from build123d import *

# Parameters (mm, degrees)
BOSS_EXTRUDE1_DEPTH = 184.15
FILLET1_R           = 3.175
FILLET2_R           = 6.35
SKETCH2_R           = 2.4638
CUT_EXTRUDE1_DEPTH  = 39.1
SKETCH3_R           = 2.4638
CUT_EXTRUDE2_DEPTH  = 39.1
LPATTERN1_COUNT     = 4
LPATTERN1_PITCH     = 101.6


with BuildPart() as part:
    # Sketch1 → Boss-Extrude1 (new body, symmetric)
    with BuildSketch(Plane(origin=(0, 0, 0), x_dir=(0, 0, -1), z_dir=(1, 0, 0))):
        Polygon((0, 38.1), (0, 0), (-38.1, 0), (-38.1, 3.175), (-3.175, 3.175), (-3.175, 38.1), align=None)
    extrude(amount=BOSS_EXTRUDE1_DEPTH, both=True)

    # Fillet1
    fillet1_edges = [part.edges().sort_by_distance(p)[0] for p in [
        (0, 3.175, 3.175),
    ]]
    fillet(fillet1_edges, radius=FILLET1_R)

    # Fillet2
    fillet2_edges = [part.edges().sort_by_distance(p)[0] for p in [
        (0, 0, 0),
    ]]
    fillet(fillet2_edges, radius=FILLET2_R)

    # Sketch2 → Cut-Extrude1 (cut, through all)
    with BuildSketch(Plane(origin=(0, 0, 0), x_dir=(-1, 0, 0), z_dir=(0, 0, -1))):
        with Locations((152.4, 19.05)):
            Circle(SKETCH2_R)
    cut_extrude1 = extrude(amount=-CUT_EXTRUDE1_DEPTH, mode=Mode.SUBTRACT)

    # Sketch3 → Cut-Extrude2 (cut, through all)
    with BuildSketch(Plane.XZ):
        with Locations((-152.4, 19.05)):
            Circle(SKETCH3_R)
    cut_extrude2 = extrude(amount=-CUT_EXTRUDE2_DEPTH, mode=Mode.SUBTRACT)

    # LPattern1: Cut-Extrude1, Cut-Extrude2 ×4
    with Locations(*[(i * LPATTERN1_PITCH, 0, 0) for i in range(1, LPATTERN1_COUNT)]):
        add(cut_extrude1, mode=Mode.SUBTRACT)
        add(cut_extrude2, mode=Mode.SUBTRACT)


solid = part.part
Can you work these out from the model? Positions are in its coordinate system, mm. A direction names the side the tool comes from. Coordinates: 2 decimals unless noted, no trailing zeros. Order: outer loops, then holes, each group sorted by start corner. A loop starts at its lowest first (then second) coordinate and runs counter-clockwise, first axis right, second up. Notation, with made-up numbers: (-26.5, 48.25) - (20.5, 48.25) arc R20 ccw to (20.5, 56.25) - close; hole circle Ø4 at (-20, 65.5). An arc over 180 degrees is marked (long way). Answer as a JSON object with one key per item and string values. Group by question number.
Q1. On a 3-axis mill with a long thin cutter (end or side, diameter ignored), from which of +Z, -Z, +X, -X, +Y, -Y can I reach the whole of each face in a straight line? I mean faces 1 (the face through (3, 3.175, 22)), 2 (the face through (-2.58, 1.81, 1.91)). Say none if no direction works.
Q2. Imagine slicing it at B-B (z = 11.5). Please give me the cut outline in (x, y) (3 decimals), and give its area (3 significant figures).
Q3. I need wall thicknesses on line 1 (X direction, y = 19, z = 2); line 2 (Y direction, x = 1, z = 20) (3 decimals); line 3 (X direction, y = 2.5, z = 18). Which ranges of each line are inside material? Lowest first, please. Write a range as from..to.
Q4. Imagine slicing it at A-A (x = 95.5). Please give me the cut outline in (y, z) (3 decimals), and give its area (3 significant figures).
Q5. Will these pins go through, and if not, where does the flat tip stop? P1, Ø6.5, axis at x = 152.4, y = 19.05, coming from the +Z side (3 decimals); P2, Ø6.5, axis at x = 152.4, z = 19.05, coming from the +Y side (3 decimals); P3, Ø4.5, axis at x = 50.8, y = 19.05, coming from the +Z side.
Determined:
{
 "1": {"face 1": "+Z, +X, -X, +Y", "face 2": "-Z, +X, -X, -Y"},
 "2": {"outline": "(-184.15, 0) - (184.15, 0) - (184.15, 3.175) - (-184.15, 3.175) - close", "area": "1,170 mm2"},
 "3": {"line 1": "x = -184.15..-154.86, -149.94..-53.26, -48.34..48.34, 53.26..149.94, 154.86..184.15", "line 2": "y = 0..3.175", "line 3": "x = -184.15..-154.63, -150.17..-53.03, -48.57..48.57, 53.03..150.17, 154.63..184.15"},
 "4": {"outline": "(0, 6.35) arc R6.35 ccw to (6.35, 0) - (38.1, 0) - (38.1, 3.175) - (6.35, 3.175) arc R3.175 cw to (3.175, 6.35) - (3.175, 38.1) - (0, 38.1) - close", "area": "225 mm2"},
 "5": {"P1": "stops at z = 3.175", "P2": "stops at y = 3.175", "P3": "passes through"}
}
